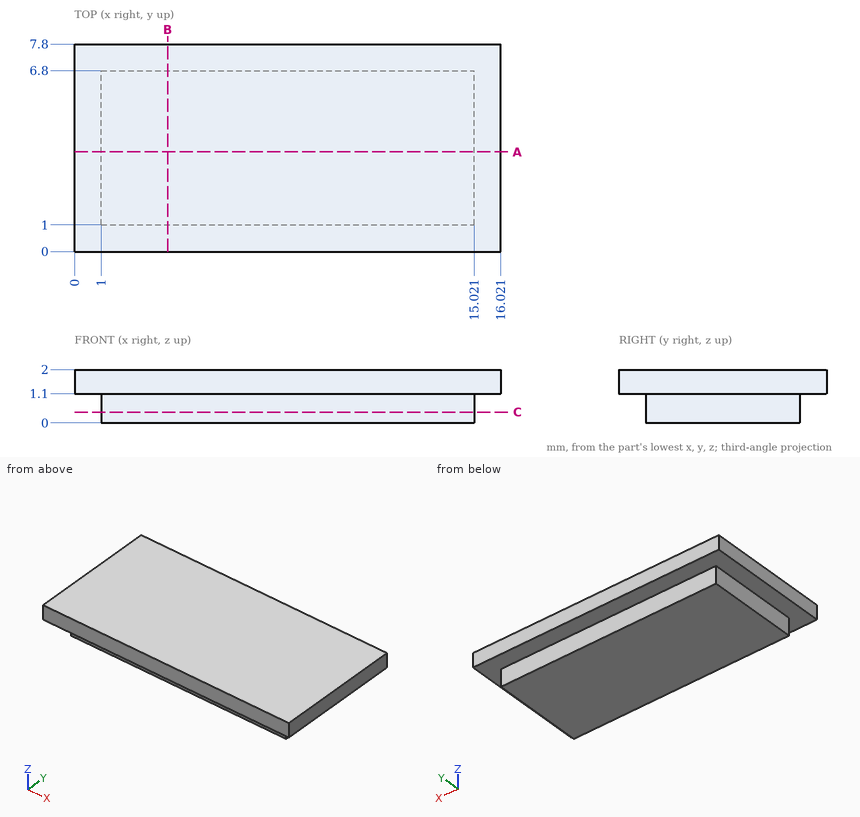
Answer from the drawing. Dimensions are ordinates in mm from the lowest x, y and z of the part. Coordinates: 2 decimals unless noted, no trailing zeros. Order: outer loops, then holes, each group sorted by start corner. A loop starts at its lowest first (then second) coordinate and runs counter-clockwise, first axis right, second up. Notation, with made-up numbers: (18.25, 11) - (76.25, 11) arc R21 ccw to (76.25, 28) - close; hole circle Ø9 at (-13, 42). An arc over 180 degrees is marked (long way). Answer as a JSON object with one key per item and string values. Group by question number.
Item 1: Section C-C (z = 0.4) is taken. Give the vertices of the cut face in (x, y), plus the area to 3 significant figures.
Item 2: Section B-B (x = 3.5) is taken. Give the vertices of the cut face in (y, z).
Item 3: Section A-A (y = 3.75) is taken. Give the vertices of the cut face in (x, z).
Item 4: Consider probe 1 along Y at (x, z) = (6.25, 0.4); probe 2 along Z at (x, y) = (12, 7.5); probe 3 along X at (y, z) = (2.25, 0.1). Determine where each line is inside the solid, lowest interval first. Write a range as from..to.
Results are:
{
 "1": {"outline": "(1, 1) - (15.02, 1) - (15.02, 6.8) - (1, 6.8) - close", "area": "81.3 mm^2"},
 "2": {"outline": "(0, 1.1) - (1, 1.1) - (1, 0) - (6.8, 0) - (6.8, 1.1) - (7.8, 1.1) - (7.8, 2) - (0, 2) - close"},
 "3": {"outline": "(0, 1.1) - (1, 1.1) - (1, 0) - (15.02, 0) - (15.02, 1.1) - (16.02, 1.1) - (16.02, 2) - (0, 2) - close"},
 "4": {"probe 1": "y = 1..6.8", "probe 2": "z = 1.1..2", "probe 3": "x = 1..15.02"}
}
